Verification items for this drawing (mm, ordinates from the low corner). A direction names the side the tool comes from. Round coordinates to 2 decimals unless told otherwise and drop trailing zeros. Order: outer loops, then holes, each group sorted by start corner. A loop starts at its lowest first (then second) coordinate and runs counter-clockwise, first axis right, second up. Notation, with made-up numbers: (-16, 19) -> (19, 19) arc R24 ccw to (19, 53) -> close; hole circle Ø2 at (11.5, -10). An arc over 180 degrees is marked (long way). Put each result on its own line as item: value.
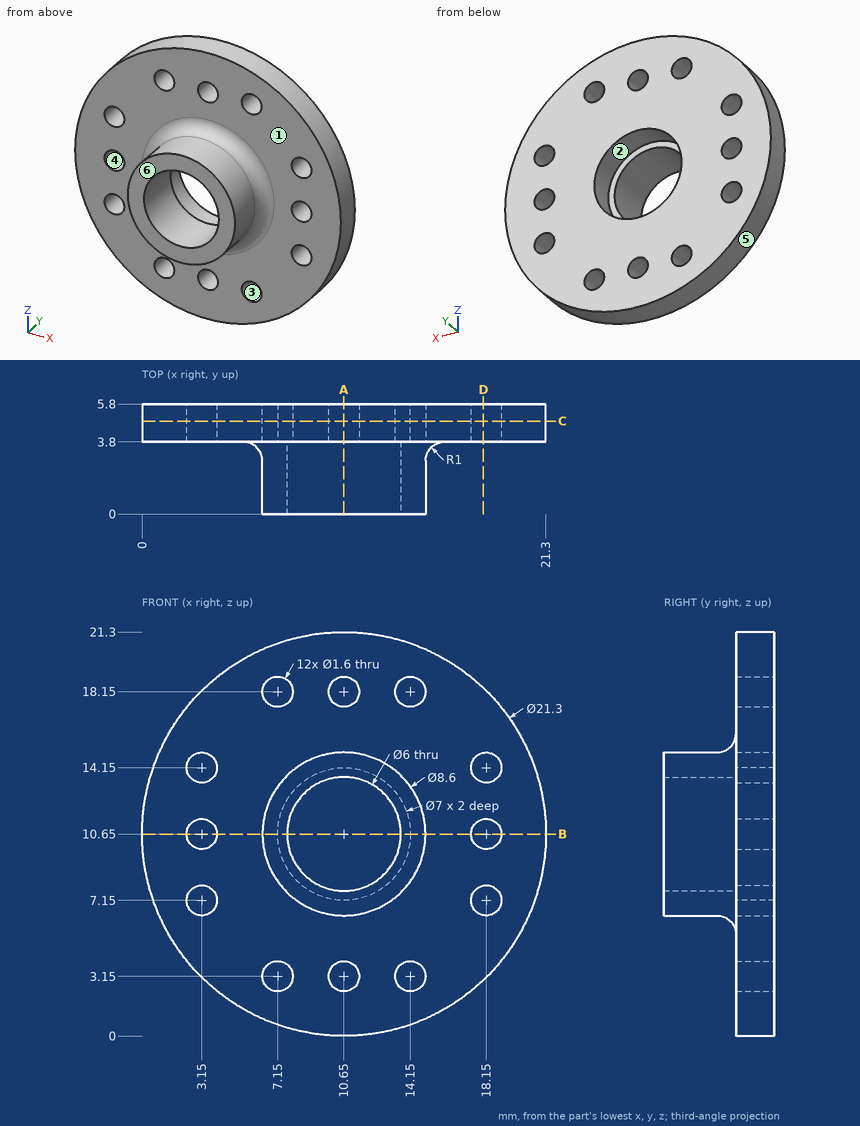
Item 1: Material ranges on L1, parallel to X at y = 5.3, z = 10.65; L2, parallel to Z at x = 18.15, y = 4.75, recorded low to high. Write a range as [from, to].
Check sheet entries:
L1: x = [0, 2.35], [3.95, 7.15], [14.15, 17.35], [18.95, 21.3]
L2: z = [3.09, 6.35], [7.95, 9.85], [11.45, 13.35], [14.95, 18.21]
Item 2: Section check A-A on x = 10.65. Record the boundary of the cut face in (y, z).
Check sheet entries:
outline: (0, 6.35) -> (2.8, 6.35) arc R1 cw to (3.8, 5.35) -> (3.8, 3.95) -> (5.8, 3.95) -> (5.8, 7.15) -> (3.8, 7.15) -> (3.8, 7.65) -> (0, 7.65) -> close; (0, 13.65) -> (3.8, 13.65) -> (3.8, 14.15) -> (5.8, 14.15) -> (5.8, 17.35) -> (3.8, 17.35) -> (3.8, 15.95) arc R1 cw to (2.8, 14.95) -> (0, 14.95) -> close; (3.8, 0) -> (5.8, 0) -> (5.8, 2.35) -> (3.8, 2.35) -> close; (3.8, 18.95) -> (5.8, 18.95) -> (5.8, 21.3) -> (3.8, 21.3) -> close
Item 3: Section check D-D on x = 18. Record the boundary of the cut face in (y, z), then the cut area to 3 significant figures.
Check sheet entries:
outline: (3.8, 2.94) -> (5.8, 2.94) -> (5.8, 6.36) -> (3.8, 6.36) -> close; (3.8, 7.94) -> (5.8, 7.94) -> (5.8, 9.86) -> (3.8, 9.86) -> close; (3.8, 11.44) -> (5.8, 11.44) -> (5.8, 13.36) -> (3.8, 13.36) -> close; (3.8, 14.94) -> (5.8, 14.94) -> (5.8, 18.36) -> (3.8, 18.36) -> close
area: 21.4 mm^2
Item 4: Section check B-B on z = 10.65. Record the boundary of the cut face in (x, y).
Check sheet entries:
outline: (0, 3.8) -> (2.35, 3.8) -> (2.35, 5.8) -> (0, 5.8) -> close; (3.95, 3.8) -> (5.35, 3.8) arc R1 cw to (6.35, 2.8) -> (6.35, 0) -> (7.65, 0) -> (7.65, 3.8) -> (7.15, 3.8) -> (7.15, 5.8) -> (3.95, 5.8) -> close; (13.65, 0) -> (14.95, 0) -> (14.95, 2.8) arc R1 cw to (15.95, 3.8) -> (17.35, 3.8) -> (17.35, 5.8) -> (14.15, 5.8) -> (14.15, 3.8) -> (13.65, 3.8) -> close; (18.95, 3.8) -> (21.3, 3.8) -> (21.3, 5.8) -> (18.95, 5.8) -> close
Item 5: Release check for a two-part mould opening along X. For the marked faces 4, 5 and 6 record: +X half, -X half, draft (parallel to the pull), parting line (faces both ways), or undercut.
Check sheet entries:
face 4: undercut
face 5: parting line
face 6: draft
Item 6: Gauge pin test, flat ends, axial feed: pin 1 Ø1 at (y, z) = (1, 10) entering from -X; pin 2 Ø2 at (x, y) = (11.5, 2.5) entering from -Z; pin 3 Ø3 at (x, y) = (5.5, 2.5) entering from -Z. Record the tip position at first contact, or that the pin passes through.
Check sheet entries:
pin 1: stops at x = 6.35
pin 2: stops at z = 6.13
pin 3: stops at z = 0.95
Item 7: Tool access check on the marked faces 1, 2 and 3. Record the directions out of +Z, -Z, +X, -X, +Y, -Y that give a thin tool (end or side, any length) a straight path to the whole face; none if there is none.
Check sheet entries:
face 1: -Y
face 2: +Y
face 3: +Y, -Y
Item 8: Section check C-C on y = 4.9. State how many separate pieces and enclosed holes the cut face has, then the cut area to 3 significant figures.
Check sheet entries:
separate pieces: 1
enclosed holes: 13
area: 294 mm^2
